Can you work these out from the model? Positions are in its coordinate system, mm. A direction names the side the tool comes from. Round coordinates to 2 decimals unless told otherwise and drop trailing zeros. Loops run counter-clockwise (first coordinate to the right, second up) from the corner with the lowest first, then second, coordinate; pieces in that order, holes last.
from build123d import *

# Parameters (mm, degrees)
SKETCH1_R           = 8.81
BOSS_EXTRUDE1_DEPTH = 15
SKETCH2_W           = 5
SKETCH2_H           = 4
BOSS_EXTRUDE2_DEPTH = 4.5
FILLET7_R           = 2
SKETCH3_R           = 1.5
CUT_EXTRUDE1_DEPTH  = 25.202937838


with BuildPart() as part:
    # Sketch1 → Boss-Extrude1 (new body)
    with BuildSketch(Plane.XY):
        Circle(SKETCH1_R)
    extrude(amount=BOSS_EXTRUDE1_DEPTH)

    # Sketch2 → Boss-Extrude2 (add)
    with BuildSketch(Plane.XY.offset(15)):
        Rectangle(SKETCH2_W, SKETCH2_H)
    extrude(amount=BOSS_EXTRUDE2_DEPTH)

    # Fillet7
    fillet7_edges = [part.edges().sort_by_distance(p)[0] for p in [
        (0, 2, 19.5),
        (0, -2, 19.5),
    ]]
    fillet(fillet7_edges, radius=FILLET7_R - 0.0001)  # a hair under: the kernel refuses the full size

    # Sketch3 → Cut-Extrude1 (cut, through all)
    with BuildSketch(Plane(origin=(2.5, 0, 0), x_dir=(0, 0, -1), z_dir=(1, 0, 0))):
        with Locations((-17.5, 0)):
            Circle(SKETCH3_R)
    extrude(amount=-CUT_EXTRUDE1_DEPTH, mode=Mode.SUBTRACT)


solid = part.part
(1) If we section it at C-C, the plane z = 9: List the corners of the cut face in (x, y) for me, then the cut area to 3 significant figures.
Worked answers:
outline: circle Ø17.62 at (0, 0)
area: 244 mm2
(2) If I drill on line 1 (Y direction, x = 1.35, z = 17.5); line 2 (Z direction, x = 3.25, y = -4.75); line 3 (Z direction, x = 2.25, y = -0.75), over which ranges is the centre line in solid material (lowest first)?
Worked answers:
line 1: y = -2 to -1.5, 1.5 to 2
line 2: z = 0 to 15
line 3: z = 0 to 16.2, 18.8 to 19.35
(3) If we section it at A-A, the plane y = -1: List the corners of the cut face in (x, z) for me.
Worked answers:
outline: (-8.75, 0) - (8.75, 0) - (8.75, 15) - (2.5, 15) - (2.5, 16.38) - (-2.5, 16.38) - (-2.5, 15) - (-8.75, 15) - close; (-2.5, 18.62) - (2.5, 18.62) - (2.5, 19.23) - (-2.5, 19.23) - close
(4) If we section it at D-D, the plane y = 4.5: List the corners of the cut face in (x, z) for me.
Worked answers:
outline: (-7.57, 0) - (7.57, 0) - (7.57, 15) - (-7.57, 15) - close
(5) For faces 4 (the flat face through (0, -2, 16)), 5 (the flat face through (-2.5, -1, 16)), 6 (the flat face through (2.5, -1, 16)), which set-ups out of +Z, -Z, +X, -X, +Y, -Y let a thin tool reach every point of the face, with its end or its side?
Worked answers:
face 4: +Z, +X, -X, -Y
face 5: +Z, -X, +Y, -Y
face 6: +Z, +X, +Y, -Y
(6) Will these pins go through, and if not, where does the flat tip stop? P1, Ø1, axis at y = 4, z = 6.5, coming from the -X side; P2, Ø10, axis at y = 6, z = 3, coming from the -X side; P3, Ø4.5, axis at y = 0.5, z = 17.5, coming from the -X side.
Worked answers:
P1: stops at x = -8.08
P2: stops at x = -8.75
P3: stops at x = -2.5
(7) If we mould it in two halves opening along Y, with no side actions, what happens to faces 1 (the cylindrical face through (0, 0, 19)), 2 (the flat face through (0, 0, 0)), 3 (the cylindrical face through (0.04, 1.43, 18.9))? For each: released by +Y, released by -Y, zero draft, split by the parting line, or undercut.
Worked answers:
face 1: undercut
face 2: zero draft
face 3: released by +Y
